Read the model definition and answer for the solid it produces. Units are mm, in the model's axes. Face numbers are marked on the shaded views. A direction names the side the tool comes from. Coordinates: 2 decimals unless noted, no trailing zeros. Loops run counter-clockwise (first coordinate to the right, second up) from the corner with the lowest first, then second, coordinate; pieces in that order, holes last. Notation, with made-up numbers: (30.5, -38) - (39.5, -38) arc R24 cw to (39.5, -19) - close; hole circle Ø8 at (-29, -12). An arc over 180 degrees is marked (long way). One line per question, with ' | ' between items. Start each with the question number.
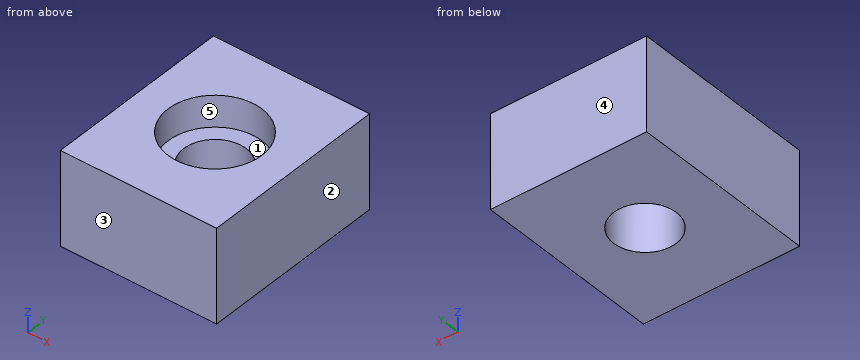
```python
from build123d import *

# Parameters (mm, degrees)
ESQUISSE1_W             = 50
ESQUISSE1_H             = 60
ESQUISSE1_R             = 10
BOSS_EXTRU_1_DEPTH      = 30
ESQUISSE2_R             = 15
ENL_V_MAT_EXTRU_1_DEPTH = 10


with BuildPart() as part:
    # Esquisse1 → Boss.-Extru.1 (new body)
    with BuildSketch(Plane.XY):
        Rectangle(ESQUISSE1_W, ESQUISSE1_H)
        Circle(ESQUISSE1_R, mode=Mode.SUBTRACT)
    extrude(amount=BOSS_EXTRU_1_DEPTH)

    # Esquisse2 → Enlèv. mat.-Extru.1 (cut)
    with BuildSketch(Plane.XY.offset(30)):
        Circle(ESQUISSE2_R)
    extrude(amount=-ENL_V_MAT_EXTRU_1_DEPTH, mode=Mode.SUBTRACT)


solid = part.part
```
1) The mould has two halves that part along X. Classify the marked faces 1, 2 and 3: released by +X, released by -X, zero draft, split by the parting line, or undercut.
2) Which of the six approach directions +Z, -Z, +X, -X, +Y, -Y give full straight-line access (tool end or side, diameter ignored) to the marked faces 4 and 5?
3) Given pin 1 Ø15 at (x, y) = (-0.5, 0.5) entering from +Z; pin 2 Ø1.5 at (x, y) = (15.5, -15) entering from -Z, each flat-ended and moving along its own axis, determine where each tip first touches the part or whether it passes through.
4) The part is cut by section D-D on y = 14. Write down the section's boundary in (x, z), and give its area (3 significant figures).
5) The part is cut by section C-C on y = 0. Write down the section's boundary in (x, z).
6) The part is cut by section B-B on x = 0. Write down the section's boundary in (y, z).
7) Find the intervals of material crossed by line 1 along X through (y, z) = (0, 10.25); line 2 along Y through (x, z) = (0, 23); line 3 along Z through (x, y) = (10.5, -10), in increasing order. Write a range as from..to.
8) The part is cut by section A-A on z = 21.75. Write down the section's boundary in (x, y), and give its area (3 significant figures).
Answer below:
1) face 1: undercut | face 2: released by +X | face 3: zero draft
2) face 4: +Z, -Z, +X, -X, +Y | face 5: +Z
3) pin 1: through | pin 2: z = 0
4) outline: (-25, 0) - (25, 0) - (25, 30) - (5.39, 30) - (5.39, 20) - (-5.39, 20) - (-5.39, 30) - (-25, 30) - close | area: 1,390 mm2
5) outline: (-25, 0) - (-10, 0) - (-10, 20) - (-15, 20) - (-15, 30) - (-25, 30) - close; (10, 0) - (25, 0) - (25, 30) - (15, 30) - (15, 20) - (10, 20) - close
6) outline: (-30, 0) - (-10, 0) - (-10, 20) - (-15, 20) - (-15, 30) - (-30, 30) - close; (10, 0) - (30, 0) - (30, 30) - (15, 30) - (15, 20) - (10, 20) - close
7) line 1: -25..-10, 10..25 | line 2: -30..-15, 15..30 | line 3: 0..20
8) outline: (-25, -30) - (25, -30) - (25, 30) - (-25, 30) - close; hole circle Ø30 at (0, 0) | area: 2,290 mm2
